```python
from build123d import *

# Parameters (mm, degrees)
F1_DEPTH = 19.05
F3_DEPTH = 19.051
F5_DEPTH = 19.051


with BuildPart() as f1:
    # F0 (on Front) → F1 (new body)
    with BuildSketch(Plane.XZ):
        with BuildLine():
            Line((660.4, 304.8), (-660.4, 304.8))
            ThreePointArc((-660.4, 304.8), (-732.242049, 275.042049), (-762, 203.2))
            Line((-762, 203.2), (-762, -914.4))
            Line((-762, -914.4), (762, -914.4))
            Line((762, -914.4), (762, 203.2))
            ThreePointArc((762, 203.2), (732.242049, 275.042049), (660.4, 304.8))
        make_face()
    extrude(amount=F1_DEPTH)

    # F2 (on face) → F3 (cut, through all)
    with BuildSketch(Plane.XZ.offset(19.05)):
        with BuildLine():
            Line((-731.379947, -127), (-744.079947, -127))
            ThreePointArc((-744.079947, -127), (-757.550331, -121.420384), (-763.129947, -107.95))
            Line((-763.129947, -107.95), (-763.129947, -50.8))
            Line((-763.129947, -50.8), (-839.329947, -50.8))
            Line((-839.329947, -50.8), (-839.329947, -431.8))
            Line((-839.329947, -431.8), (-763.129947, -431.8))
            Line((-763.129947, -431.8), (-763.129947, -381))
            ThreePointArc((-763.129947, -381), (-748.250971, -345.078976), (-712.329947, -330.2))
            Line((-712.329947, -330.2), (-693.279947, -330.2))
            Line((-693.279947, -330.2), (-693.279947, -50.8))
            Line((-693.279947, -50.8), (-712.329947, -50.8))
            Line((-712.329947, -50.8), (-712.329947, -107.95))
            ThreePointArc((-712.329947, -107.95), (-717.909562, -121.420384), (-731.379947, -127))
        make_face()
        with BuildLine():
            Line((-712.329947, -457.2), (-712.329947, -514.35))
            ThreePointArc((-712.329947, -514.35), (-717.909562, -527.820384), (-731.379947, -533.4))
            Line((-731.379947, -533.4), (-744.079947, -533.4))
            ThreePointArc((-744.079947, -533.4), (-757.550331, -527.820384), (-763.129947, -514.35))
            Line((-763.129947, -514.35), (-763.129947, -457.2))
            Line((-763.129947, -457.2), (-839.329947, -457.2))
            Line((-839.329947, -457.2), (-839.329947, -838.2))
            Line((-839.329947, -838.2), (-763.129947, -838.2))
            Line((-763.129947, -838.2), (-763.129947, -787.4))
            ThreePointArc((-763.129947, -787.4), (-748.250971, -751.478976), (-712.329947, -736.6))
            Line((-712.329947, -736.6), (-693.279947, -736.6))
            Line((-693.279947, -736.6), (-693.279947, -457.2))
            Line((-693.279947, -457.2), (-712.329947, -457.2))
        make_face()
        with BuildLine():
            ThreePointArc((763.129947, -107.95), (757.550331, -121.420384), (744.079947, -127))
            Line((744.079947, -127), (731.379947, -127))
            ThreePointArc((731.379947, -127), (717.909562, -121.420384), (712.329947, -107.95))
            Line((712.329947, -107.95), (712.329947, -50.8))
            Line((712.329947, -50.8), (693.279947, -50.8))
            Line((693.279947, -50.8), (693.279947, -330.2))
            Line((693.279947, -330.2), (712.329947, -330.2))
            ThreePointArc((712.329947, -330.2), (748.250971, -345.078976), (763.129947, -381))
            Line((763.129947, -381), (763.129947, -431.8))
            Line((763.129947, -431.8), (839.329947, -431.8))
            Line((839.329947, -431.8), (839.329947, -50.8))
            Line((839.329947, -50.8), (763.129947, -50.8))
            Line((763.129947, -50.8), (763.129947, -107.95))
        make_face()
        with BuildLine():
            Line((693.279947, -457.2), (693.279947, -736.6))
            Line((693.279947, -736.6), (712.329947, -736.6))
            ThreePointArc((712.329947, -736.6), (748.250971, -751.478976), (763.129947, -787.4))
            Line((763.129947, -787.4), (763.129947, -838.2))
            Line((763.129947, -838.2), (839.329947, -838.2))
            Line((839.329947, -838.2), (839.329947, -457.2))
            Line((839.329947, -457.2), (763.129947, -457.2))
            Line((763.129947, -457.2), (763.129947, -514.35))
            ThreePointArc((763.129947, -514.35), (757.550331, -527.820384), (744.079947, -533.4))
            Line((744.079947, -533.4), (731.379947, -533.4))
            ThreePointArc((731.379947, -533.4), (717.909562, -527.820384), (712.329947, -514.35))
            Line((712.329947, -514.35), (712.329947, -457.2))
            Line((712.329947, -457.2), (693.279947, -457.2))
        make_face()
    extrude(amount=-F3_DEPTH, mode=Mode.SUBTRACT)

    # F4 (on face) → F5 (cut, through all)
    with BuildSketch(Plane.XZ.offset(19.05)):
        with BuildLine():
            ThreePointArc((-50.8, 152.346021), (-68.760512, 144.906534), (-76.2, 126.946021))
            Line((-76.2, 126.946021), (-76.2, -711.253979))
            ThreePointArc((-76.2, -711.253979), (-68.760512, -729.214491), (-50.8, -736.653979))
            ThreePointArc((-50.8, -736.653979), (-32.839488, -729.214491), (-25.4, -711.253979))
            Line((-25.4, -711.253979), (-25.4, 126.946021))
            ThreePointArc((-25.4, 126.946021), (-32.839488, 144.906534), (-50.8, 152.346021))
        make_face()
        with BuildLine():
            ThreePointArc((-152.4, 152.346021), (-170.360512, 144.906534), (-177.8, 126.946021))
            Line((-177.8, 126.946021), (-177.8, -711.253979))
            ThreePointArc((-177.8, -711.253979), (-170.360512, -729.214491), (-152.4, -736.653979))
            ThreePointArc((-152.4, -736.653979), (-134.439488, -729.214491), (-127, -711.253979))
            Line((-127, -711.253979), (-127, 126.946021))
            ThreePointArc((-127, 126.946021), (-134.439488, 144.906534), (-152.4, 152.346021))
        make_face()
        with BuildLine():
            ThreePointArc((-254, 152.346021), (-271.960512, 144.906534), (-279.4, 126.946021))
            Line((-279.4, 126.946021), (-279.4, -711.253979))
            ThreePointArc((-279.4, -711.253979), (-271.960512, -729.214491), (-254, -736.653979))
            ThreePointArc((-254, -736.653979), (-236.039488, -729.214491), (-228.6, -711.253979))
            Line((-228.6, -711.253979), (-228.6, 126.946021))
            ThreePointArc((-228.6, 126.946021), (-236.039488, 144.906534), (-254, 152.346021))
        make_face()
        with BuildLine():
            ThreePointArc((-355.6, 152.346021), (-373.560512, 144.906534), (-381, 126.946021))
            Line((-381, 126.946021), (-381, -711.253979))
            ThreePointArc((-381, -711.253979), (-373.560512, -729.214491), (-355.6, -736.653979))
            ThreePointArc((-355.6, -736.653979), (-337.639488, -729.214491), (-330.2, -711.253979))
            Line((-330.2, -711.253979), (-330.2, 126.946021))
            ThreePointArc((-330.2, 126.946021), (-337.639488, 144.906534), (-355.6, 152.346021))
        make_face()
        with BuildLine():
            ThreePointArc((-457.2, 152.346021), (-475.160512, 144.906534), (-482.6, 126.946021))
            Line((-482.6, 126.946021), (-482.6, -711.253979))
            ThreePointArc((-482.6, -711.253979), (-475.160512, -729.214491), (-457.2, -736.653979))
            ThreePointArc((-457.2, -736.653979), (-439.239488, -729.214491), (-431.8, -711.253979))
            Line((-431.8, -711.253979), (-431.8, 126.946021))
            ThreePointArc((-431.8, 126.946021), (-439.239488, 144.906534), (-457.2, 152.346021))
        make_face()
        with BuildLine():
            ThreePointArc((-558.8, 152.346021), (-576.760512, 144.906534), (-584.2, 126.946021))
            Line((-584.2, 126.946021), (-584.2, -711.253979))
            ThreePointArc((-584.2, -711.253979), (-576.760512, -729.214491), (-558.8, -736.653979))
            ThreePointArc((-558.8, -736.653979), (-540.839488, -729.214491), (-533.4, -711.253979))
            Line((-533.4, -711.253979), (-533.4, 126.946021))
            ThreePointArc((-533.4, 126.946021), (-540.839488, 144.906534), (-558.8, 152.346021))
        make_face()
        with BuildLine():
            ThreePointArc((127, -711.253979), (134.439488, -729.214491), (152.4, -736.653979))
            ThreePointArc((152.4, -736.653979), (170.360512, -729.214491), (177.8, -711.253979))
            Line((177.8, -711.253979), (177.8, 126.946021))
            ThreePointArc((177.8, 126.946021), (170.360512, 144.906534), (152.4, 152.346021))
            ThreePointArc((152.4, 152.346021), (134.439488, 144.906534), (127, 126.946021))
            Line((127, 126.946021), (127, -711.253979))
        make_face()
        with BuildLine():
            ThreePointArc((482.6, 126.946021), (475.160512, 144.906534), (457.2, 152.346021))
            ThreePointArc((457.2, 152.346021), (439.239488, 144.906534), (431.8, 126.946021))
            Line((431.8, 126.946021), (431.8, -711.253979))
            ThreePointArc((431.8, -711.253979), (439.239488, -729.214491), (457.2, -736.653979))
            ThreePointArc((457.2, -736.653979), (475.160512, -729.214491), (482.6, -711.253979))
            Line((482.6, -711.253979), (482.6, 126.946021))
        make_face()
        with BuildLine():
            ThreePointArc((254, -736.653979), (271.960512, -729.214491), (279.4, -711.253979))
            Line((279.4, -711.253979), (279.4, 126.946021))
            ThreePointArc((279.4, 126.946021), (271.960512, 144.906534), (254, 152.346021))
            ThreePointArc((254, 152.346021), (236.039488, 144.906534), (228.6, 126.946021))
            Line((228.6, 126.946021), (228.6, -711.253979))
            ThreePointArc((228.6, -711.253979), (236.039488, -729.214491), (254, -736.653979))
        make_face()
        with BuildLine():
            ThreePointArc((558.8, 152.346021), (540.839488, 144.906534), (533.4, 126.946021))
            Line((533.4, 126.946021), (533.4, -711.253979))
            ThreePointArc((533.4, -711.253979), (540.839488, -729.214491), (558.8, -736.653979))
            ThreePointArc((558.8, -736.653979), (576.760512, -729.214491), (584.2, -711.253979))
            Line((584.2, -711.253979), (584.2, 126.946021))
            ThreePointArc((584.2, 126.946021), (576.760512, 144.906534), (558.8, 152.346021))
        make_face()
        with BuildLine():
            ThreePointArc((355.6, 152.346021), (337.639488, 144.906534), (330.2, 126.946021))
            Line((330.2, 126.946021), (330.2, -711.253979))
            ThreePointArc((330.2, -711.253979), (337.639488, -729.214491), (355.6, -736.653979))
            ThreePointArc((355.6, -736.653979), (373.560512, -729.214491), (381, -711.253979))
            Line((381, -711.253979), (381, 126.946021))
            ThreePointArc((381, 126.946021), (373.560512, 144.906534), (355.6, 152.346021))
        make_face()
        with BuildLine():
            ThreePointArc((25.4, -711.253979), (32.839488, -729.214491), (50.8, -736.653979))
            ThreePointArc((50.8, -736.653979), (68.760512, -729.214491), (76.2, -711.253979))
            Line((76.2, -711.253979), (76.2, 126.946021))
            ThreePointArc((76.2, 126.946021), (68.760512, 144.906534), (50.8, 152.346021))
            ThreePointArc((50.8, 152.346021), (32.839488, 144.906534), (25.4, 126.946021))
            Line((25.4, 126.946021), (25.4, -711.253979))
        make_face()
    extrude(amount=-F5_DEPTH, mode=Mode.SUBTRACT)


solid = f1.part
```
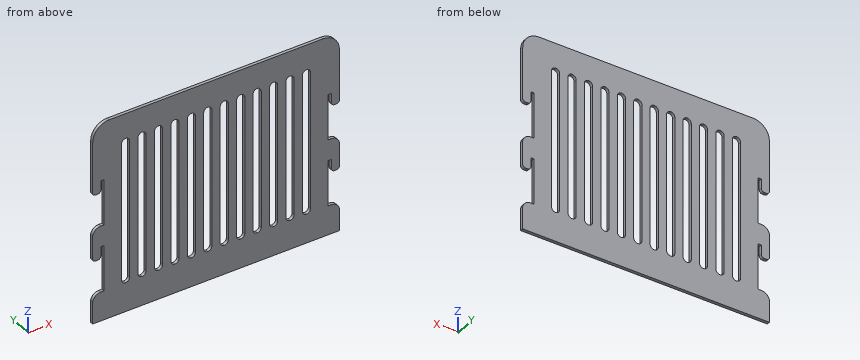
CAD build for the part. Positions are in the model's coordinates, mm. Round coordinates to 2 decimals unless told otherwise and drop trailing zeros. Answer in a Markdown table with one row per item. Add a question column.
(1) Drop flat-ended pins along their axis: pin 1 Ø5.5 at (y, z) = (-13, -194.5) entering from -X; pin 2 Ø1 at (y, z) = (-13, -758) entering from -X; pin 3 Ø5.5 at (y, z) = (-10, -120) entering from -X. Give the stop position or say it passes through.
(2) Band-saw the part on A-A on y = -14.25. Count the separate pieces of the cut face and the enclosed holes in it, and give its area (3 significant figures).
(3) Probe L1, parallel to Z at x = -150, y = -5.5; L2, parallel to Z at x = 555, y = -8.25; L3, parallel to X at y = -17.25, z = 230.5. List the from-to ranges inside material, lowest first. Write a range as [from, to].
Data:
| question | item | result |
|---|---|---|
| 1 | pin 1 | stops at x = -693.28 |
| 1 | pin 2 | stops at x = -754.11 |
| 1 | pin 3 | stops at x = -760.71 |
| 2 | separate pieces | 1 |
| 2 | enclosed holes | 12 |
| 2 | area | 1,250,000 mm^2 |
| 3 | L1 | z = [-914.4, -736.54], [152.23, 304.8] |
| 3 | L2 | z = [-914.4, -736.37], [152.06, 304.8] |
| 3 | L3 | x = [-758.26, 758.26] |
